The listing builds one solid part. Answer for the finished solid, in the listing's coordinates (mm). A direction names the side the tool comes from. Coordinates: 2 decimals unless noted, no trailing zeros. Write each loop counter-clockwise with the first axis right and the second up, starting at its lowest first coordinate (ties: lowest second). Pieces come first, ordered by that corner, then holes.
from build123d import *

# Parameters (mm, degrees)
SKETCH_1_R      = 1
EXTRUDE_1_DEPTH = 0.5
EXTRUDE1_START  = -0.5
EXTRUDE1_DEPTH  = 1
EXTRUDE2_DEPTH  = 0.5
FILLET1_R       = 1.6
FILLET2_R       = 3.2


# Read off the part's stored shape, not the designer's step: Extrude1
with BuildPart() as part:
    # Эскиз1 → Бобышка-Вытянуть1 (new, symmetric)
    with BuildSketch(Plane.XY):
        with BuildLine():
            Line((0, 2), (-28.5003, 2))
            ThreePointArc((-28.5003, 2), (-30.5003, 0), (-28.5003, -2))
            Line((-28.5003, -2), (0, -2))
            ThreePointArc((0, -2), (2, 0), (0, 2))
        make_face()
        with Locations((-28.5003, 0)):
            Circle(SKETCH_1_R, mode=Mode.SUBTRACT)
        Circle(SKETCH_1_R, mode=Mode.SUBTRACT)
    extrude(amount=EXTRUDE_1_DEPTH, both=True)

    # Extrude1 outline → Extrude1 (add)
    with BuildSketch(Plane.XY.offset(EXTRUDE1_START)):
        with BuildLine():
            ThreePointArc((-9.154212394, 2), (-13.9, 5.15), (-18.645787606, 2))
            Line((-18.645787606, 2), (-9.154212394, 2))
        make_face()
    extrude(amount=EXTRUDE1_DEPTH)

    # Sketch → Extrude2 (cut, symmetric)
    with BuildSketch(Plane.XY):
        with BuildLine():
            ThreePointArc((-11.879660865, 0.735343308), (-12.140166364, 1.235105491), (-12.521595125, 1.65))
            Line((-12.521595125, 1.65), (-15.278404875, 1.65))
            ThreePointArc((-15.278404875, 1.65), (-15.659833636, 1.235105491), (-15.920339135, 0.735343308))
            Line((-15.920339135, 0.735343308), (-16.915922679, -2))
            Line((-16.915922679, -2), (-10.884077321, -2))
            Line((-10.884077321, -2), (-11.879660865, 0.735343308))
        make_face()
        with BuildLine():
            ThreePointArc((-11.686405638, 4.65), (-13.9, 5.15), (-16.113594362, 4.65))
            Line((-16.113594362, 4.65), (-11.686405638, 4.65))
        make_face()
    extrude(amount=EXTRUDE2_DEPTH, both=True, mode=Mode.SUBTRACT)

    # Fillet1
    fillet1_edges = [part.edges().sort_by_distance(p)[0] for p in [
        (-18.645787606, 2, 0),
        (-9.154212394, 2, 0),
        (-15.278404875, 1.65, 0),
        (-12.521595125, 1.65, 0),
    ]]
    fillet(fillet1_edges, radius=FILLET1_R)

    # Fillet2
    fillet2_edges = [part.edges().sort_by_distance(p)[0] for p in [
        (-10.884077321, -2, 0),
        (-16.915922679, -2, 0),
        (-11.686405638, 4.65, 0),
        (-16.113594362, 4.65, 0),
    ]]
    fillet(fillet2_edges, radius=FILLET2_R)


solid = part.part
Q1. Given pin 1 (1.6 mm diameter, centred on x = 0, y = 0, fed in from +Z); pin 2 (0.5 mm diameter, centred on x = -2, z = 0, fed in from +Y), each flat-ended and moving along its own axis, determine where each tip first touches the part or whether it passes through.
Answers below:
pin 1: passes through
pin 2: stops at y = 2
Q2. The part is cut by section B-B, the plane x = -0.5. Write down the section's boundary in (y, z).
Answers below:
outline: (-2, -0.5) - (-0.87, -0.5) - (-0.87, 0.5) - (-2, 0.5) - close; (0.87, -0.5) - (2, -0.5) - (2, 0.5) - (0.87, 0.5) - close
Q3. Which of the six approach directions +Z, -Z, +X, -X, +Y, -Y give full straight-line access (tool end or side, diameter ignored) to faces 5 (the face through (-4, 2, 0)), 6 (the face through (-17.299, -1.405, -0.007)), 7 (the face through (-14, 2, -0.5)), 8 (the face through (-24, 2, 0))?
Answers below:
face 5: +Z, -Z, +X, +Y
face 6: +Z, -Z, -Y
face 7: -Z, +X, -X, +Y, -Y
face 8: +Z, -Z, -X, +Y
Q4. Determine the mould class of faces 1 (the face through (-14, 1.65, 0)), 2 (the face through (0, -1, 0)), 3 (the face through (2, 0, 0)), 4 (the face through (-18.85, 2.19, 0.01)) for opening direction X: released by +X, released by -X, zero draft, split by the parting line, or undercut.
Answers below:
face 1: undercut
face 2: undercut
face 3: released by +X
face 4: released by -X
Q5. The part is cut by section A-A, the plane y = -0.5. Write down the section's boundary in (x, z), then the cut area to 3 significant figures.
Answers below:
outline: (-30.44, -0.5) - (-29.37, -0.5) - (-29.37, 0.5) - (-30.44, 0.5) - close; (-27.63, -0.5) - (-16.45, -0.5) - (-16.45, 0.5) - (-27.63, 0.5) - close; (-11.35, -0.5) - (-0.87, -0.5) - (-0.87, 0.5) - (-11.35, 0.5) - close; (0.87, -0.5) - (1.94, -0.5) - (1.94, 0.5) - (0.87, 0.5) - close
area: 23.8 mm2
Q6. The part is cut by section C-C, the plane z = -0.2. State how many separate pieces and enclosed holes the cut face has, then the cut area to 3 significant figures.
Answers below:
separate pieces: 1
enclosed holes: 2
area: 122 mm2
Q7. The part is cut by section D-D, the plane x = -5.5. Write down the section's boundary in (y, z).
Answers below:
outline: (-2, -0.5) - (2, -0.5) - (2, 0.5) - (-2, 0.5) - close
Q8. Find the intervals of material crossed by probe 1 along X at (y, z) = (-0.75, 0); probe 2 along Y at (x, z) = (-20, 0); probe 3 along X at (y, z) = (1.5, 0.4), in increasing order.
Answers below:
probe 1: x = -30.35 to -29.16, -27.84 to -16.62, -11.18 to -0.66, 0.66 to 1.85
probe 2: y = -2 to 2
probe 3: x = -29.82 to -15.14, -12.66 to 1.32
